For this review, take the finished solid that the model builds, in its own axes (mm). Face numbers are marked on the shaded views. A direction names the side the tool comes from. Give positions to 0.01 mm unless a question says otherwise; leave off trailing zeros. Write each loop counter-clockwise with the first axis right and the second up, starting at its lowest first coordinate (ties: lowest second). Pieces come first, ordered by that corner, then holes. Notation, with made-up numbers: (57, -2) -> (101, -2) arc R4 cw to (101, 5) -> close; hole circle Ø10 at (-31, 42). An arc over 180 degrees is marked (long way). Return JSON: item names as keys, results as strings.
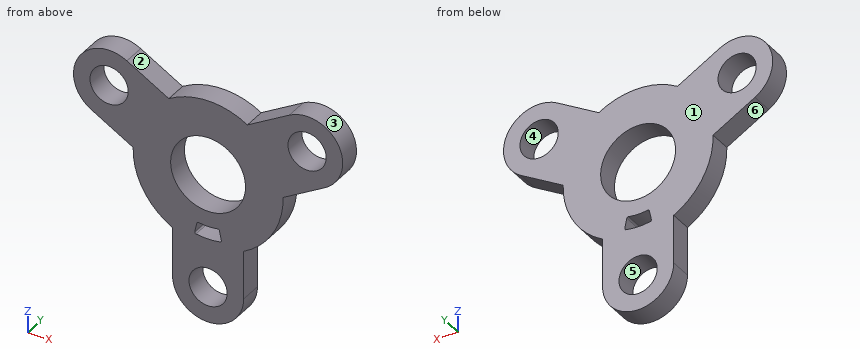
from build123d import *

# Parameters (mm, degrees)
SKETCH1_R           = 10
SKETCH1_R_2         = 5
BOSS_EXTRUDE1_DEPTH = 3
BOSS_EXTRUDE2_START = -3
SKETCH2_R           = 2.55
BOSS_EXTRUDE2_DEPTH = 3
CIRPATTERN1_COUNT   = 3
CUT_EXTRUDE1_DEPTH  = 28.045328716
FILLET1_R           = 0.2


with BuildPart() as part:
    # Sketch1 → Boss-Extrude1 (new body)
    with BuildSketch(Plane(origin=(0, 0, 0), x_dir=(1, 0, 0), z_dir=(0, 1, 0))):
        with Locations(Location((0, 0, 0), (0, 0, 270))):
            Circle(SKETCH1_R)
        with Locations(Location((0, 0, 0), (0, 0, 270))):
            Circle(SKETCH1_R_2, mode=Mode.SUBTRACT)
    extrude(amount=BOSS_EXTRUDE1_DEPTH)

    # Sketch2 → Boss-Extrude2 (add)
    with BuildSketch(Plane(origin=(0, 3, 0), x_dir=(1, 0, 0), z_dir=(0, 1, 0)).offset(BOSS_EXTRUDE2_START)):
        with BuildLine():
            Line((-4.75, 15.25), (-4.75, 8.799857953))
            ThreePointArc((-4.75, 8.799857953), (0, 10), (4.75, 8.799857953))
            Line((4.75, 8.799857953), (4.75, 15.25))
            ThreePointArc((4.75, 15.25), (0, 20), (-4.75, 15.25))
        make_face()
        with Locations(Location((0, 15.25, 0), (0, 0, 270))):
            Circle(SKETCH2_R, mode=Mode.SUBTRACT)
    boss_extrude2 = extrude(amount=BOSS_EXTRUDE2_DEPTH)

    # CirPattern1: Boss-Extrude2 ×3 about axis
    cirpattern1_axis = Axis((0, 0, 0), (0, 1, 0))
    for i in range(1, CIRPATTERN1_COUNT):
        add(boss_extrude2.rotate(cirpattern1_axis, i * 360 / CIRPATTERN1_COUNT))

    # Sketch3 → Cut-Extrude1 (cut, through all)
    with BuildSketch(Plane(origin=(0, 3, 0), x_dir=(1, 0, 0), z_dir=(0, 1, 0))):
        with BuildLine():
            Line((-1.819227295, 8.558791506), (-1.46577742, 6.895940585))
            ThreePointArc((-1.46577742, 6.895940585), (0, 7.05), (1.46577742, 6.895940585))
            Line((1.46577742, 6.895940585), (1.819227295, 8.558791506))
            ThreePointArc((1.819227295, 8.558791506), (0, 8.75), (-1.819227295, 8.558791506))
        make_face()
    extrude(amount=-CUT_EXTRUDE1_DEPTH, mode=Mode.SUBTRACT)

    # Fillet1
    fillet1_edges = [part.edges().sort_by_distance(p)[0] for p in [
        (1.46577742, 1.5, -6.895940585),
        (-1.46577742, 1.5, -6.895940585),
        (-1.819227295, 1.5, -8.558791506),
        (1.819227295, 1.5, -8.558791506),
    ]]
    fillet(fillet1_edges, radius=FILLET1_R)


solid = part.part
1. Add section A-A, the plane x = 0. State the section outline as (y, z) points, plus the area to 3 significant figures.
Results found:
{"outline": "(0, -20) -> (3, -20) -> (3, -17.8) -> (0, -17.8) -> close; (0, -12.7) -> (3, -12.7) -> (3, -8.75) -> (0, -8.75) -> close; (0, -7.05) -> (3, -7.05) -> (3, -5) -> (0, -5) -> close; (0, 5) -> (3, 5) -> (3, 10) -> (0, 10) -> close", "area": "39.6 mm²"}
2. For pin 1 (0.9 mm diameter, centred on y = 2, z = -13, fed in from -X); pin 2 (1.5 mm diameter, centred on y = 2.5, z = 6, fed in from +X), all flat-tipped, find the tip position at first contact; note any pin that passes through.
Results found:
{"pin 1": "stops at x = -4.75", "pin 2": "stops at x = 17.88"}
3. For the marked faces 1 and 2, list the 3-axis set-ups (+Z, -Z, +X, -X, +Y, -Y) from which the entire face can be reached by the end or side of a thin tool; tool diameter is ignored.
Results found:
{"face 1": "+Z, -Z, +X, -X, +Y", "face 2": "+Z, +Y, -Y"}
4. To check wall thickness, follow probe 1 along X at (y, z) = (0.9, 0); probe 2 along X at (y, z) = (2.3, 7); probe 3 along X at (y, z) = (0.6, -15.25). State the ranges of each line that lie inside material, in increasing order.
Results found:
{"probe 1": "x = -10 to -5, 5 to 10", "probe 2": "x = -17.92 to -15.68, -10.73 to 10.73, 15.68 to 17.92", "probe 3": "x = -4.75 to -2.55, 2.55 to 4.75"}
5. Add section B-B, the plane z = -3.5. State the section outline as (x, y) points, plus the area to 3 significant figures.
Results found:
{"outline": "(-9.37, 0) -> (-3.57, 0) -> (-3.57, 3) -> (-9.37, 3) -> close; (3.57, 0) -> (9.37, 0) -> (9.37, 3) -> (3.57, 3) -> close", "area": "34.8 mm²"}
6. Add section C-C, the plane z = 8. State the section outline as (x, y) points, plus the area to 3 significant figures.
Results found:
{"outline": "(-17.94, 0) -> (-15.73, 0) -> (-15.73, 3) -> (-17.94, 3) -> close; (-10.68, 0) -> (10.68, 0) -> (10.68, 3) -> (-10.68, 3) -> close; (15.73, 0) -> (17.94, 0) -> (17.94, 3) -> (15.73, 3) -> close", "area": "77.4 mm²"}
7. The part is to be moulded in two halves that separate along Z. For the marked faces 3, 4, 5 and 6, say which applies: +Z half, -Z half, draft (parallel to the pull), parting line (faces both ways), or undercut.
Results found:
{"face 3": "parting line", "face 4": "undercut", "face 5": "undercut", "face 6": "-Z half"}
8. Add section D-D, the plane x = -12.5. State the section outline as (y, z) points, plus the area to 3 significant figures.
Results found:
{"outline": "(0, 1.73) -> (3, 1.73) -> (3, 5.17) -> (0, 5.17) -> close; (0, 10.08) -> (3, 10.08) -> (3, 12.32) -> (0, 12.32) -> close", "area": "17.1 mm²"}
